Autodesk Inventor part; units mm, degrees
ref_plane "YZ Plane" through (0, 0, 0) normal (1, 0, 0) x (0, 1, 0)
ref_plane "XZ Plane" through (0, 0, 0) normal (0, 1, 0) x (-1, 0, 0)
ref_plane "XY Plane" through (0, 0, 0) normal (0, 0, 1) x (1, 0, 0)
sketch "Sketch1" plane through (0, 0, 0) normal (0, 1, 0) x (-1, 0, 0)
  line L0 (2, 0) -> (39.392, 0)
  line L1 (41.392, -2) -> (41.392, -80)
  line L2 (39.392, -82) -> (2, -82)
  line L3 (0, -80) -> (0, -2)
  arc A0 (41.392, -2) -> (39.392, 0) centre (39.392, -2) ccw
  arc A1 (39.392, -82) -> (41.392, -80) centre (39.392, -80) ccw
  arc A2 (0, -80) -> (2, -82) centre (2, -80) ccw
  arc A3 (2, 0) -> (0, -2) centre (2, -2) ccw
  circle A4 centre (39.386, -2.006) radius 1.1
  circle A5 centre (39.386, -79.994) radius 1.1
  circle A6 centre (2.006, -2.006) radius 1.1
  circle A7 centre (2.006, -79.994) radius 1.1
  point P0 (0, 0)
  point P1 (41.392, -82)
  point P2 (41.392, 0)
  point P3 (0, -82)
  dimension "d0" = 41.392
  dimension "d1" = 82
  dimension "d2" = 2
  dimension "d3" = 2.2
  dimension "d5" = 2.006
  dimension "d6" = 2.006
  dimension "d7" = 2.2
  dimension "d8" = 2.006
  dimension "d9" = 2.006
  dimension "d10" = 2.2
  dimension "d11" = 2.006
  dimension "d12" = 2.006
  dimension "d13" = 2.2
  dimension "d14" = 2.006
  dimension "d15" = 2.006
  dimension "d16" = 37.386
extrude "Extrusion1" add sketch "Sketch1" along normal blind 1.5
properties part number "battery_cover"
For this review, take the finished solid that the model builds, in its own axes (mm). Give positions to 0.01 mm unless a question says otherwise; leave off trailing zeros. Answer as a JSON object with one key per item and string values. Group by question number.
Item 1: For pin 1 Ø2 at (x, z) = (-29.5, -66) entering from -Y; pin 2 Ø1.3 at (x, z) = (-2.006, -79.994) entering from -Y, all flat-tipped, find the tip position at first contact; note any pin that passes through.
Item 2: For probe 1 along Z at (x, y) = (-39, 0.9), list the stretches that pass through material, from the lowest coordinate up. Write a range as [from, to].
Item 3: Draft analysis for pull direction X (two halves, no side actions). For faces 1 (the cylindrical face through (-0.6, 0.74, -81.43)), 2 (the cylindrical face through (-40.82, 0.74, -81.4)), 3 (the cylindrical face through (-38.58, 0.74, -80.74)), state which applies: +X half, -X half, draft (parallel to the pull), parting line (faces both ways), or undercut.
Check result:
{
 "1": {"pin 1": "stops at y = 0", "pin 2": "passes through"},
 "2": {"probe 1": "z = [-82, -81.02], [-78.96, -3.04], [-0.98, 0]"},
 "3": {"face 1": "+X half", "face 2": "-X half", "face 3": "undercut"}
}
